Here's how the part is built. I have some questions about the finished solid (model axes, mm). A direction names the side the tool comes from. Round coordinates to 2 decimals unless told otherwise and drop trailing zeros. Use one line per item in the form item = value. Start each with the question number.
1. If I drill on line 1 along Y through (x, z) = (235, 0.95); line 2 along Y through (x, z) = (226.5, 1.65); line 3 along Y through (x, z) = (230, 2.1), over which ranges is the centre line in solid material (lowest first)?
2. I want a section at A-A, the plane z = 1. State how many separate pieces and enclosed holes the cut face has, plus the area to 3 significant figures.
3. We'd pull the mould along X, two halves only. Please class faces 1 (the cylindrical face through (234.93, -211.82, 1.48)), 2 (the flat face through (229, -85.217, 1)), 3 (the flat face through (222.453, -79, 1)): +X half, -X half, draft (parallel to the pull), parting line (faces both ways), or undercut.
4. Which directions (+Z, -Z, +X, -X, +Y, -Y) give clear straight access to the entire face, cutting with the end or side of a thin tool? Please do faces 4 (the flat face through (222.453, -211, 1)), 5 (the flat face through (271, -195.037, 1)), 6 (the flat face through (229, -198.037, 1)).
5. Will these pins go through, and if not, where does the flat tip stop? pin 1 (0.9 mm diameter, centred on x = 229, z = 1, fed in from -Y); pin 2 (0.9 mm diameter, centred on x = 229.5, z = 2, fed in from -Y); pin 3 (1.5 mm diameter, centred on y = -84, z = 1, fed in from -X).
```python
from build123d import *

# Parameters (mm, degrees)
SKETCH_1_R      = 5.5
SKETCH_1_R_2    = 2
EXTRUDE_1_DEPTH = 3


with BuildPart() as part:
    # 草图1 → 凸台-拉伸1 (new body)
    with BuildSketch(Plane.XY):
        with BuildLine():
            Line((222.453360513, -82.216557036), (222.453360513, -75.216557036))
            Line((222.453360513, -75.216557036), (277.453360513, -75.216557036))
            Line((277.453360513, -75.216557036), (277.453360513, -82.216557036))
            Line((277.453360513, -82.216557036), (274.953360513, -82.216557036))
            Line((274.953360513, -82.216557036), (274.953360513, -80.716557036))
            Line((274.953360513, -80.716557036), (272.353360513, -80.716557036))
            Line((272.353360513, -80.716557036), (272.353360513, -82.216557036))
            Line((272.353360513, -82.216557036), (269.353360513, -82.216557036))
            Line((269.353360513, -82.216557036), (269.353360513, -85.216557036))
            Line((269.353360513, -85.216557036), (272.353360513, -85.216557036))
            Line((272.353360513, -85.216557036), (272.353360513, -86.716557036))
            Line((272.353360513, -86.716557036), (274.953360513, -86.716557036))
            Line((274.953360513, -86.716557036), (274.953360513, -85.216557036))
            Line((274.953360513, -85.216557036), (277.453360513, -85.216557036))
            Line((277.453360513, -85.216557036), (277.453360513, -195.037068397))
            Line((277.453360513, -195.037068397), (274.953360513, -195.037068397))
            Line((274.953360513, -195.037068397), (274.953360513, -193.537068397))
            Line((274.953360513, -193.537068397), (272.353360513, -193.537068397))
            Line((272.353360513, -193.537068397), (272.353360513, -195.037068397))
            Line((272.353360513, -195.037068397), (269.353360513, -195.037068397))
            Line((269.353360513, -195.037068397), (269.353360513, -198.037068397))
            Line((269.353360513, -198.037068397), (272.353360513, -198.037068397))
            Line((272.353360513, -198.037068397), (272.353360513, -199.537068397))
            Line((272.353360513, -199.537068397), (274.953360513, -199.537068397))
            Line((274.953360513, -199.537068397), (274.953360513, -198.037068397))
            Line((274.953360513, -198.037068397), (277.453360513, -198.037068397))
            Line((277.453360513, -198.037068397), (277.453360513, -224.037068397))
            ThreePointArc((277.453360513, -224.037068397), (249.953360513, -251.537068397), (222.453360513, -224.037068397))
            Line((222.453360513, -224.037068397), (222.453360513, -198.037068397))
            Line((222.453360513, -198.037068397), (224.953360513, -198.037068397))
            Line((224.953360513, -198.037068397), (224.953360513, -199.537068397))
            Line((224.953360513, -199.537068397), (227.553360513, -199.537068397))
            Line((227.553360513, -199.537068397), (227.553360513, -198.037068397))
            Line((227.553360513, -198.037068397), (230.553360513, -198.037068397))
            Line((230.553360513, -198.037068397), (230.553360513, -195.037068397))
            Line((230.553360513, -195.037068397), (227.553360513, -195.037068397))
            Line((227.553360513, -195.037068397), (227.553360513, -193.537068397))
            Line((227.553360513, -193.537068397), (224.953360513, -193.537068397))
            Line((224.953360513, -193.537068397), (224.953360513, -195.037068397))
            Line((224.953360513, -195.037068397), (222.453360513, -195.037068397))
            Line((222.453360513, -195.037068397), (222.453360513, -85.216557036))
            Line((222.453360513, -85.216557036), (224.953360513, -85.216557036))
            Line((224.953360513, -85.216557036), (224.953360513, -86.716557036))
            Line((224.953360513, -86.716557036), (227.553360513, -86.716557036))
            Line((227.553360513, -86.716557036), (227.553360513, -85.216557036))
            Line((227.553360513, -85.216557036), (230.553360513, -85.216557036))
            Line((230.553360513, -85.216557036), (230.553360513, -82.216557036))
            Line((230.553360513, -82.216557036), (227.553360513, -82.216557036))
            Line((227.553360513, -82.216557036), (227.553360513, -80.716557036))
            Line((227.553360513, -80.716557036), (224.953360513, -80.716557036))
            Line((224.953360513, -80.716557036), (224.953360513, -82.216557036))
            Line((224.953360513, -82.216557036), (222.453360513, -82.216557036))
        make_face()
        with Locations((249.953360513, -224.037068397)):
            Circle(SKETCH_1_R, mode=Mode.SUBTRACT)
        with Locations((249.953360513, -205.037068397)):
            Circle(SKETCH_1_R_2, mode=Mode.SUBTRACT)
        with Locations((263.388389356, -210.602039555)):
            Circle(SKETCH_1_R_2, mode=Mode.SUBTRACT)
        with Locations((268.953360513, -224.037068397)):
            Circle(SKETCH_1_R_2, mode=Mode.SUBTRACT)
        with Locations((263.388389356, -237.47209724)):
            Circle(SKETCH_1_R_2, mode=Mode.SUBTRACT)
        with Locations((249.953360513, -243.037068397)):
            Circle(SKETCH_1_R_2, mode=Mode.SUBTRACT)
        with Locations((236.518331671, -237.47209724)):
            Circle(SKETCH_1_R_2, mode=Mode.SUBTRACT)
        with Locations((230.953360513, -224.037068397)):
            Circle(SKETCH_1_R_2, mode=Mode.SUBTRACT)
        with Locations((236.518331671, -210.602039555)):
            Circle(SKETCH_1_R_2, mode=Mode.SUBTRACT)
    extrude(amount=EXTRUDE_1_DEPTH)


solid = part.part
```
Model answer:
q1.line_1 = -247.12 to -238.77, -236.17 to -211.9, -209.3 to -75.22
q1.line_2 = -238.4 to -199.54, -193.54 to -86.72, -80.72 to -75.22
q1.line_3 = -242.96 to -225.8, -222.28 to -198.04, -195.04 to -85.22, -82.22 to -75.22
q2.separate_pieces = 1
q2.enclosed_holes = 9
q2.area = 9,050 mm2
q3.face_1 = undercut
q3.face_2 = draft
q3.face_3 = -X half
q4.face_4 = +Z, -Z, -X, +Y, -Y
q4.face_5 = +Z, -Z, +X
q4.face_6 = +Z, -Z, -X
q5.pin_1 = -242.36
q5.pin_2 = -242.91
q5.pin_3 = 230.55
